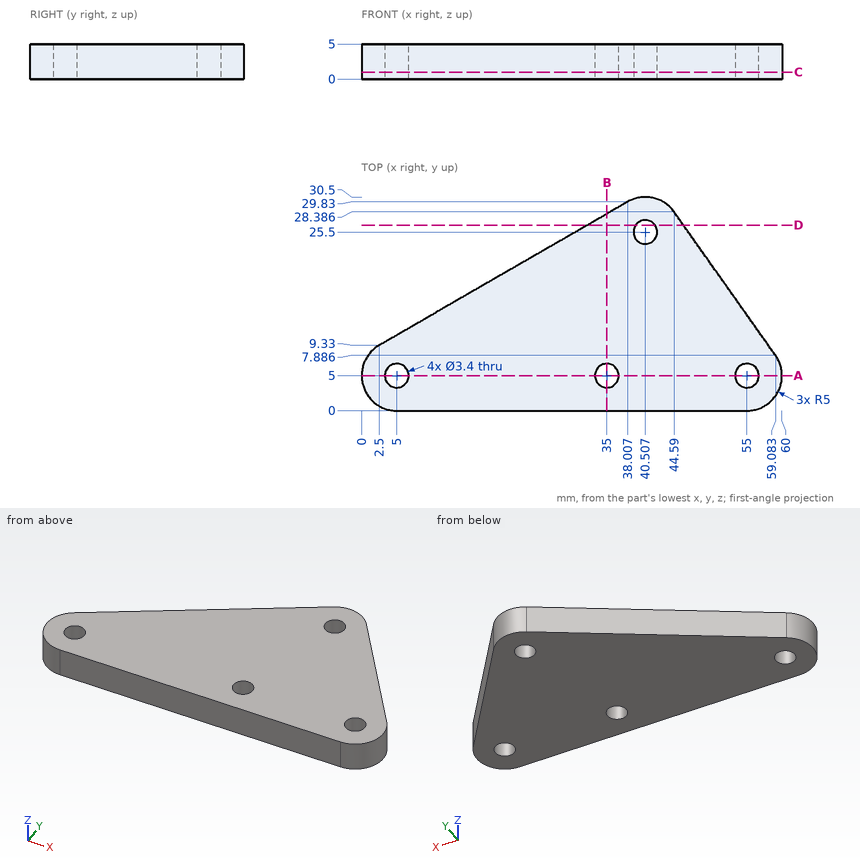
For this review, use the dimensioned drawing (mm, ordinates from the lowest corner) and the shaded views. Round coordinates to 2 decimals unless told otherwise and drop trailing zeros. Loops run counter-clockwise (first coordinate to the right, second up) from the corner with the lowest first, then second, coordinate; pieces in that order, holes last. Notation, with made-up numbers: M -26.75,42 L 8.25,42 A9 cw 8.25,55 Z; hole C 64,63 d4. An arc over 180 degrees is marked long. Answer as a JSON object with one key per item and string values.
(1) Clearance check with a flat-ended pin moving along its axis: P1, Ø3, axis at x = 40.51, y = 25.5, coming from the -Z side. State where the tip first meets the part, or that it passes through.
Resolved:
{"P1": "through"}
(2) To check wall thickness, follow line 1 along X through (y, z) = (4, 4.3) (1 decimal); line 2 along Y through (x, z) = (5.5, 3) (1 decimal); line 3 along Y through (x, z) = (56, 1.75) (1 decimal). State the ranges of each line that lie inside material, in increasing order.
Resolved:
{"line 1": "0.1 to 3.6, 6.4 to 33.6, 36.4 to 53.6, 56.4 to 59.9", "line 2": "0 to 3.4, 6.6 to 11.1", "line 3": "0.1 to 3.6, 6.4 to 12.2"}
(3) Take a section at D-D on y = 26.5. Give the boundary of the cut face in (x, z).
Resolved:
{"outline": "M 32.24,0 L 39.13,0 L 39.13,5 L 32.24,5 Z; M 41.88,0 L 45.92,0 L 45.92,5 L 41.88,5 Z"}
(4) Take a section at C-C on z = 1. Give the boundary of the cut face in (x, y).
Resolved:
{"outline": "M 2.5,9.33 A5 ccw 5,0 L 55,0 A5 ccw 59.08,7.89 L 44.59,28.39 A5 ccw 38.01,29.83 Z; hole C 5,5 d3.4; hole C 35,5 d3.4; hole C 40.51,25.5 d3.4; hole C 55,5 d3.4"}
(5) Take a section at B-B on x = 35. Give the boundary of the cut face in (y, z).
Resolved:
{"outline": "M 0,0 L 3.3,0 L 3.3,5 L 0,5 Z; M 6.7,0 L 28.09,0 L 28.09,5 L 6.7,5 Z"}
(6) Take a section at A-A on y = 5. Give the boundary of the cut face in (x, z), and give its area (3 significant figures).
Resolved:
{"outline": "M 0,0 L 3.3,0 L 3.3,5 L 0,5 Z; M 6.7,0 L 33.3,0 L 33.3,5 L 6.7,5 Z; M 36.7,0 L 53.3,0 L 53.3,5 L 36.7,5 Z; M 56.7,0 L 60,0 L 60,5 L 56.7,5 Z", "area": "249 mm²"}
